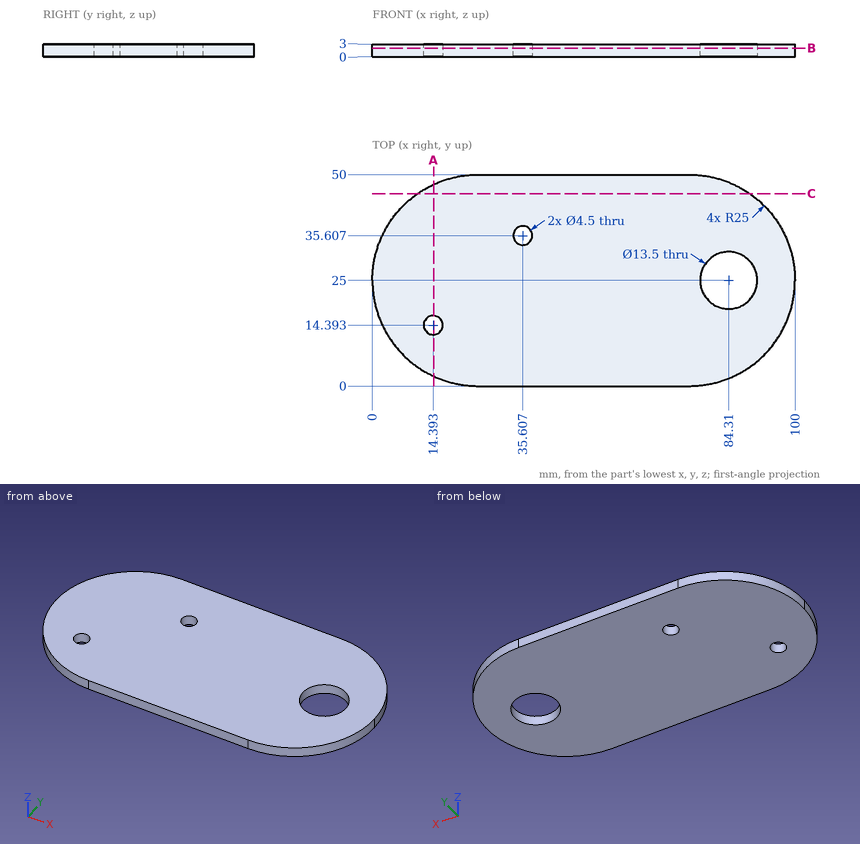
Study the drawing (mm; zero at the part's minimum x, y, z) and answer. Coordinates: 2 decimals unless noted, no trailing zeros. Loops run counter-clockwise (first coordinate to the right, second up) from the corner with the lowest first, then second, coordinate; pieces in that order, holes last. Notation, with made-up numbers: (83, 50.25) -> (87, 50.25) arc R20 ccw to (87, 87.25) -> close; hole circle Ø6 at (75, 55.5). An arc over 180 degrees is marked (long way). Write each question's results on one line, items separated by ' | '. Start each with the question number.
1) Find section A-A on x = 14.5. Determine the outline of the cut face in (y, z).
2) Flat-ended cylindrical pins translate along their axes: P1, Ø1, axis at y = 41, z = 0.5, coming from the +X side (1 decimal); P2, Ø12, axis at x = 84.31, y = 25, coming from the -Z side; P3, Ø8, axis at x = 24.5, y = 24.5, coming from the -Z side. Find the tip coordinate at first contact, or state that the pin passes through.
3) Find section B-B on z = 2. Count the separate pieces of the cut face and the enclosed holes in it, then the cut area to 3 significant figures.
4) Find section C-C on y = 45.5. Determine the outline of the cut face in (x, z), then the cut area to 3 significant figures.
5) Consider line 1 along Y through (x, z) = (24, 1.1); line 2 along X through (y, z) = (21, 1.2) (1 decimal); line 3 along Y through (x, z) = (82, 0.75). Determine where each line is inside the solid, lowest interval first.
Response values:
1) outline: (2.31, 0) -> (12.15, 0) -> (12.15, 3) -> (2.31, 3) -> close; (16.64, 0) -> (47.69, 0) -> (47.69, 3) -> (16.64, 3) -> close
2) P1: stops at x = 94.6 | P2: passes through | P3: stops at z = 0
3) separate pieces: 1 | enclosed holes: 3 | area: 4,290 mm^2
4) outline: (10.69, 0) -> (89.31, 0) -> (89.31, 3) -> (10.69, 3) -> close | area: 236 mm^2
5) line 1: y = 0.02 to 49.98 | line 2: x = 0.3 to 78.9, 89.7 to 99.7 | line 3: y = 1 to 18.66, 31.34 to 49
